Geometry: final body of the model. Coordinates: model frame, mm. Coordinates: 2 decimals unless noted, no trailing zeros. Order: outer loops, then holes, each group sorted by start corner. A loop starts at its lowest first (then second) coordinate and runs counter-clockwise, first axis right, second up. Notation, with made-up numbers: (62.25, 6.25) - (80.25, 6.25) arc R17 ccw to (80.25, 17.25) - close; hole circle Ø7 at (89.5, -22). An arc over 180 degrees is marked (long way). Use a Markdown table: item, result. Add a question column.
```python
from build123d import *

# Parameters (mm, degrees)
SKETCH1_W               = 203.2
SKETCH1_H               = 152.4
BOSS_EXTRUDE1_DEPTH     = 3.175
SKETCH2_W               = 12.7
SKETCH2_H               = 3.175
BOSS_EXTRUDE2_DEPTH     = 3.175
BOSS_EXTRUDE2_2_DEPTH   = 3.175
BOSS_EXTRUDE2_3_DEPTH   = 3.175
BOSS_EXTRUDE2_4_DEPTH   = 3.175
BOSS_EXTRUDE2_5_DEPTH   = 3.175
BOSS_EXTRUDE2_6_DEPTH   = 3.175
BOSS_EXTRUDE2_7_DEPTH   = 3.175
BOSS_EXTRUDE2_8_DEPTH   = 3.175
BOSS_EXTRUDE2_9_DEPTH   = 3.175
BOSS_EXTRUDE2_10_DEPTH  = 3.175
BOSS_EXTRUDE2_11_DEPTH  = 3.175
BOSS_EXTRUDE2_12_DEPTH  = 3.175
BOSS_EXTRUDE2_13_DEPTH  = 3.175
BOSS_EXTRUDE2_14_DEPTH  = 3.175
BOSS_EXTRUDE2_15_DEPTH  = 3.175
BOSS_EXTRUDE2_16_DEPTH  = 3.175
SKETCH4_R               = 2.249999945
CUT_EXTRUDE1_DEPTH      = 4.175
SKETCH5_R               = 2.249999945
CUT_EXTRUDE2_DEPTH      = 4.175
SKETCH10_R              = 2.249999945
CUT_EXTRUDE3_DEPTH      = 1
CUT_EXTRUDE3_DEPTH_BACK = 4.175
SKETCH11_W              = 6.35
SKETCH11_H              = 3.175
CUT_EXTRUDE4_DEPTH      = 4.175


with BuildPart() as part:
    # Sketch1 → Boss-Extrude1 (new body)
    with BuildSketch(Plane(origin=(0, 0, 0), x_dir=(1, 0, 0), z_dir=(0, 1, 0))):
        with Locations((101.6, 76.2)):
            Rectangle(SKETCH1_W, SKETCH1_H)
    extrude(amount=BOSS_EXTRUDE1_DEPTH)

    # Sketch4 → Cut-Extrude1 (cut, through all)
    with BuildSketch(Plane(origin=(163.318517222, 3.175, 18.128898402), x_dir=(-1, 0, 0), z_dir=(0, 1, 0))):
        with Locations((62.768517222, -41.828898402)):
            Circle(SKETCH4_R)
        with Locations((62.768517222, -90.828898402)):
            Circle(SKETCH4_R)
        with Locations((120.768517222, -90.828898402)):
            Circle(SKETCH4_R)
        with Locations((120.768517222, -41.828898402)):
            Circle(SKETCH4_R)
    extrude(amount=-CUT_EXTRUDE1_DEPTH, mode=Mode.SUBTRACT)

    # Sketch5 → Cut-Extrude2 (cut, through all)
    with BuildSketch(Plane(origin=(307.482010873, 3.175, -268.648993813), x_dir=(-1, 0, 0), z_dir=(0, 1, 0))):
        with Locations((140.407118473, 210.304081528)):
            Circle(SKETCH5_R)
        with Locations((141.507118473, 258.104081528)):
            Circle(SKETCH5_R)
        with Locations((192.307118473, 215.004081528)):
            Circle(SKETCH5_R)
        with Locations((192.307118473, 242.904081528)):
            Circle(SKETCH5_R)
    extrude(amount=-CUT_EXTRUDE2_DEPTH, mode=Mode.SUBTRACT)

    # Sketch10 → Cut-Extrude3 (cut, two sides)
    with BuildSketch(Plane(origin=(154.738240667, 3.175, -89.784200023), x_dir=(0, 0, -1), z_dir=(0, 1, 0))) as cut_extrude3_sk:
        with Locations((-3.423776116, 48.068240667)):
            Circle(SKETCH10_R)
        with Locations((52.455799977, 48.285900219)):
            Circle(SKETCH10_R)
        with Locations((-3.423776116, -38.291759333)):
            Circle(SKETCH10_R)
        with Locations((52.455799977, -38.074099781)):
            Circle(SKETCH10_R)
    extrude(amount=CUT_EXTRUDE3_DEPTH, mode=Mode.SUBTRACT)
    extrude(cut_extrude3_sk.sketch, amount=-CUT_EXTRUDE3_DEPTH_BACK, mode=Mode.SUBTRACT)


with BuildPart() as body_2:
    # Sketch2 → Boss-Extrude2 (new body)
    with BuildSketch(Plane(origin=(0, 3.175, 0), x_dir=(1, 0, 0), z_dir=(0, 1, 0))):
        with Locations((31.75, -1.5875)):
            Rectangle(SKETCH2_W, SKETCH2_H)
    extrude(amount=-BOSS_EXTRUDE2_DEPTH)


with BuildPart() as body_3:
    # Sketch2 → Boss-Extrude2 2 (new body)
    with BuildSketch(Plane(origin=(0, 3.175, 0), x_dir=(1, 0, 0), z_dir=(0, 1, 0))):
        with Locations((6.35, -1.5875)):
            Rectangle(SKETCH2_W, SKETCH2_H)
    extrude(amount=-BOSS_EXTRUDE2_2_DEPTH)


with BuildPart() as body_4:
    # Sketch2 → Boss-Extrude2 3 (new body)
    with BuildSketch(Plane(origin=(0, 3.175, 0), x_dir=(1, 0, 0), z_dir=(0, 1, 0))):
        with Locations((57.15, -1.5875)):
            Rectangle(SKETCH2_W, SKETCH2_H)
    extrude(amount=-BOSS_EXTRUDE2_3_DEPTH)


with BuildPart() as body_5:
    # Sketch2 → Boss-Extrude2 4 (new body)
    with BuildSketch(Plane(origin=(0, 3.175, 0), x_dir=(1, 0, 0), z_dir=(0, 1, 0))):
        with Locations((82.55, -1.5875)):
            Rectangle(SKETCH2_W, SKETCH2_H)
    extrude(amount=-BOSS_EXTRUDE2_4_DEPTH)


with BuildPart() as body_6:
    # Sketch2 → Boss-Extrude2 5 (new body)
    with BuildSketch(Plane(origin=(0, 3.175, 0), x_dir=(1, 0, 0), z_dir=(0, 1, 0))):
        with Locations((107.95, -1.5875)):
            Rectangle(SKETCH2_W, SKETCH2_H)
    extrude(amount=-BOSS_EXTRUDE2_5_DEPTH)


with BuildPart() as body_7:
    # Sketch2 → Boss-Extrude2 6 (new body)
    with BuildSketch(Plane(origin=(0, 3.175, 0), x_dir=(1, 0, 0), z_dir=(0, 1, 0))):
        with Locations((133.35, -1.5875)):
            Rectangle(SKETCH2_W, SKETCH2_H)
    extrude(amount=-BOSS_EXTRUDE2_6_DEPTH)


with BuildPart() as body_8:
    # Sketch2 → Boss-Extrude2 7 (new body)
    with BuildSketch(Plane(origin=(0, 3.175, 0), x_dir=(1, 0, 0), z_dir=(0, 1, 0))):
        with Locations((158.75, -1.5875)):
            Rectangle(SKETCH2_W, SKETCH2_H)
    extrude(amount=-BOSS_EXTRUDE2_7_DEPTH)


with BuildPart() as body_9:
    # Sketch2 → Boss-Extrude2 8 (new body)
    with BuildSketch(Plane(origin=(0, 3.175, 0), x_dir=(1, 0, 0), z_dir=(0, 1, 0))):
        with Locations((184.15, -1.5875)):
            Rectangle(SKETCH2_W, SKETCH2_H)
    extrude(amount=-BOSS_EXTRUDE2_8_DEPTH)


with BuildPart() as body_10:
    # Sketch2 → Boss-Extrude2 9 (new body)
    with BuildSketch(Plane(origin=(0, 3.175, 0), x_dir=(1, 0, 0), z_dir=(0, 1, 0))):
        with Locations((184.15, 153.9875)):
            Rectangle(SKETCH2_W, SKETCH2_H)
    extrude(amount=-BOSS_EXTRUDE2_9_DEPTH)


with BuildPart() as body_11:
    # Sketch2 → Boss-Extrude2 10 (new body)
    with BuildSketch(Plane(origin=(0, 3.175, 0), x_dir=(1, 0, 0), z_dir=(0, 1, 0))):
        with Locations((158.75, 153.9875)):
            Rectangle(SKETCH2_W, SKETCH2_H)
    extrude(amount=-BOSS_EXTRUDE2_10_DEPTH)


with BuildPart() as body_12:
    # Sketch2 → Boss-Extrude2 11 (new body)
    with BuildSketch(Plane(origin=(0, 3.175, 0), x_dir=(1, 0, 0), z_dir=(0, 1, 0))):
        with Locations((133.35, 153.9875)):
            Rectangle(SKETCH2_W, SKETCH2_H)
    extrude(amount=-BOSS_EXTRUDE2_11_DEPTH)


with BuildPart() as body_13:
    # Sketch2 → Boss-Extrude2 12 (new body)
    with BuildSketch(Plane(origin=(0, 3.175, 0), x_dir=(1, 0, 0), z_dir=(0, 1, 0))):
        with Locations((107.95, 153.9875)):
            Rectangle(SKETCH2_W, SKETCH2_H)
    extrude(amount=-BOSS_EXTRUDE2_12_DEPTH)


with BuildPart() as body_14:
    # Sketch2 → Boss-Extrude2 13 (new body)
    with BuildSketch(Plane(origin=(0, 3.175, 0), x_dir=(1, 0, 0), z_dir=(0, 1, 0))):
        with Locations((82.55, 153.9875)):
            Rectangle(SKETCH2_W, SKETCH2_H)
    extrude(amount=-BOSS_EXTRUDE2_13_DEPTH)


with BuildPart() as body_15:
    # Sketch2 → Boss-Extrude2 14 (new body)
    with BuildSketch(Plane(origin=(0, 3.175, 0), x_dir=(1, 0, 0), z_dir=(0, 1, 0))):
        with Locations((57.15, 153.9875)):
            Rectangle(SKETCH2_W, SKETCH2_H)
    extrude(amount=-BOSS_EXTRUDE2_14_DEPTH)


with BuildPart() as body_16:
    # Sketch2 → Boss-Extrude2 15 (new body)
    with BuildSketch(Plane(origin=(0, 3.175, 0), x_dir=(1, 0, 0), z_dir=(0, 1, 0))):
        with Locations((31.75, 153.9875)):
            Rectangle(SKETCH2_W, SKETCH2_H)
    extrude(amount=-BOSS_EXTRUDE2_15_DEPTH)


with BuildPart() as body_17:
    # Sketch2 → Boss-Extrude2 16 (new body)
    with BuildSketch(Plane(origin=(0, 3.175, 0), x_dir=(1, 0, 0), z_dir=(0, 1, 0))):
        with Locations((6.35, 153.9875)):
            Rectangle(SKETCH2_W, SKETCH2_H)
    extrude(amount=-BOSS_EXTRUDE2_16_DEPTH)


with BuildPart() as body_3_1:
    add(body_3.part)

    # Combine1: union body 4, body 6, body 8, body 10, body 12, body 14, body 16, body 17, part, body 2, body 5, body 7, body 9, body 11, body 13, body 15
    add(body_4.part)
    add(body_6.part)
    add(body_8.part)
    add(body_10.part)
    add(body_12.part)
    add(body_14.part)
    add(body_16.part)
    add(body_17.part)
    add(part.part)
    add(body_2.part)
    add(body_5.part)
    add(body_7.part)
    add(body_9.part)
    add(body_11.part)
    add(body_13.part)
    add(body_15.part)

    # Sketch11 → Cut-Extrude4 (cut, through all)
    with BuildSketch(Plane(origin=(0, 3.175, 0), x_dir=(1, 0, 0), z_dir=(0, 1, 0))):
        with Locations((8.255, 77.7875)):
            Rectangle(SKETCH11_W, SKETCH11_H)
    extrude(amount=-CUT_EXTRUDE4_DEPTH, mode=Mode.SUBTRACT)


solid = body_3_1.part
```
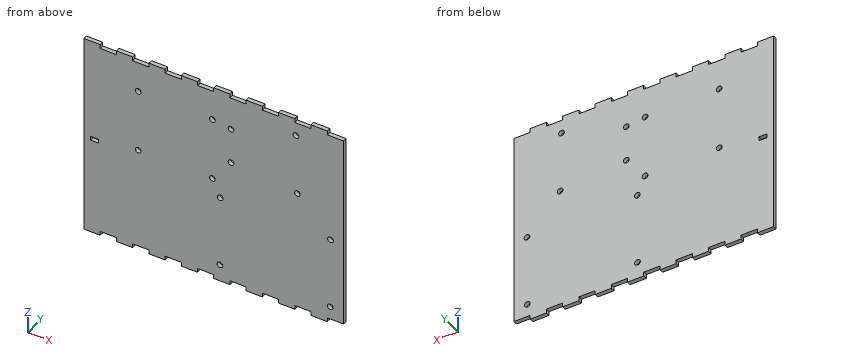
1) Section B-B (x = 42.55). Return loops of the section in (y, z) (3 decimals).
2) Pin query (flat end, axial travel): pin 1 (2 mm diameter, centred on x = 141.5, z = -47, fed in from -Y); pin 2 (3.5 mm diameter, centred on x = 100.55, z = -72.7, fed in from -Y); pin 3 (1.6 mm diameter, centred on x = 19, y = 2, fed in from -Z); pin 4 (1.5 mm diameter, centred on x = 99, y = 2, fed in from +Z). Return the tip coordinate at first contact, or that it passes through.
3) Section A-A (z = -142.24). Return loops of the section in (x, y) (3 decimals).
4) Section C-C (y = 0.55). Give the number of separate pieces and of enclosed holes in the cut face, then the cut area to 3 significant figures.
5) Ray query, line 1 along X through (y, z) = (1.65, -142.24); line 2 along Z through (x, y) = (42.55, 0.7); line 3 along X through (y, z) = (0.65, -25.5). Return the intervals inside material, ascending.
6) Section D-D (x = 172). Return loops of the section in (y, z) (3 decimals), then the cut area to 3 significant figures.
Values follow:
| question | item | result |
|---|---|---|
| 1 | outline | (0, -152.4) - (3.175, -152.4) - (3.175, -74.95) - (0, -74.95) - close; (0, -70.45) - (3.175, -70.45) - (3.175, -25.95) - (0, -25.95) - close; (0, -21.45) - (3.175, -21.45) - (3.175, 0) - (0, 0) - close |
| 2 | pin 1 | stops at y = 0 |
| 2 | pin 2 | passes through |
| 2 | pin 3 | stops at z = -152.4 |
| 2 | pin 4 | stops at z = 0 |
| 3 | outline | (0, 0) - (104.202, 0) - (104.202, 3.175) - (0, 3.175) - close; (108.702, 0) - (190.562, 0) - (190.562, 3.175) - (108.702, 3.175) - close; (195.062, 0) - (203.2, 0) - (203.2, 3.175) - (195.062, 3.175) - close |
| 4 | separate pieces | 1 |
| 4 | enclosed holes | 13 |
| 4 | area | 31,400 mm² |
| 5 | line 1 | x = 0 to 104.2, 108.7 to 190.56, 195.06 to 203.2 |
| 5 | line 2 | z = -152.4 to -74.95, -70.45 to -25.95, -21.45 to 0 |
| 5 | line 3 | x = 0 to 41.2, 43.9 to 99.2, 101.9 to 112.94, 117.41 to 203.2 |
| 6 | outline | (0, -152.4) - (3.175, -152.4) - (3.175, 0) - (0, 0) - close |
| 6 | area | 484 mm² |
